```python
from build123d import *

# Parameters (mm, degrees)
SKETCH1_W                  = 63.5
SKETCH1_H                  = 60.452
BOSS_EXTRUDE1_DEPTH        = 1.27
SKETCH2_W                  = 16.51
SKETCH2_H                  = 4.826
SKETCH2_W_2                = 38.1
SKETCH2_H_2                = 8.89
SKETCH2_H_3                = 7.62
BOSS_EXTRUDE2_DEPTH        = 15.24
SKETCH3_R                  = 1.905
CUT_EXTRUDE1_DEPTH         = 25.892
SKETCH4_R                  = 3.175
CUT_EXTRUDE2_DEPTH         = 7.62
SKETCH5_W                  = 22.86
SKETCH5_H                  = 24.252018656
SKETCH5_H_2                = 1.10530733
SKETCH5_H_3                = 10.202674014
CUT_EXTRUDE3_DEPTH         = 18.78
F_8_0_199_DIAMETER_HOLE1_D = 5.0546


with BuildPart() as part:
    # Sketch1 → Boss-Extrude1 (new body, symmetric)
    with BuildSketch(Plane(origin=(0, 0, 0), x_dir=(1, 0, 0), z_dir=(0, 1, 0))):
        Rectangle(SKETCH1_W, SKETCH1_H)
    extrude(amount=BOSS_EXTRUDE1_DEPTH, both=True)

    # Sketch2 → Boss-Extrude2 (add)
    with BuildSketch(Plane(origin=(0, 1.27, 0), x_dir=(1, 0, 0), z_dir=(0, 1, 0))):
        with Locations((-23.495, 27.813)):
            Rectangle(SKETCH2_W, SKETCH2_H)
        with Locations((-23.495, -0.889)):
            Rectangle(SKETCH2_W, SKETCH2_H)
        with Locations((0, -25.781)):
            Rectangle(SKETCH2_W_2, SKETCH2_H_2)
        with Locations((0, -9.144)):
            Rectangle(SKETCH2_W_2, SKETCH2_H_3)
    extrude(amount=BOSS_EXTRUDE2_DEPTH)

    # Sketch3 → Cut-Extrude1 (cut, through all)
    with BuildSketch(Plane(origin=(0, 0, 5.334), x_dir=(-1, 0, 0), z_dir=(0, 0, -1))):
        with Locations((1.524, 4.445)):
            Circle(SKETCH3_R)
    extrude(amount=-CUT_EXTRUDE1_DEPTH, mode=Mode.SUBTRACT)

    # Sketch4 → Cut-Extrude2 (cut)
    with BuildSketch(Plane(origin=(0, 0, 5.334), x_dir=(-1, 0, 0), z_dir=(0, 0, -1))):
        with Locations((1.524, 4.445)):
            Circle(SKETCH4_R)
    extrude(amount=-CUT_EXTRUDE2_DEPTH, mode=Mode.SUBTRACT)

    # Sketch5 → Cut-Extrude3 (cut, through all)
    with BuildSketch(Plane.XZ.offset(1.27)):
        with Locations((8.89, -16.994683342)):
            Rectangle(SKETCH5_W, SKETCH5_H)
        with Locations((8.89, -29.673346335)):
            Rectangle(SKETCH5_W, SKETCH5_H_2)
        with Locations((8.89, 0.232662993)):
            Rectangle(SKETCH5_W, SKETCH5_H_3)
    extrude(amount=-CUT_EXTRUDE3_DEPTH, mode=Mode.SUBTRACT)

    # #8 (0.199) Diameter Hole1 (through all)
    with Locations(Plane(origin=(-6.35, 1.27, 1.524), x_dir=(0, 0, 1), z_dir=(0, 1, 0))):
        with Locations((0, 0), (15.875, -12.7), (-19.05, 31.75)):
            Hole(F_8_0_199_DIAMETER_HOLE1_D / 2)


solid = part.part
```
Can you work these out from the model? Positions are in its coordinate system, mm. A direction names the side the tool comes from. Give positions to 0.01 mm unless a question says otherwise; leave off trailing zeros. Loops run counter-clockwise (first coordinate to the right, second up) from the corner with the lowest first, then second, coordinate; pieces in that order, holes last. Notation, with made-up numbers: M 21.25,-10.75 L 50.25,-10.75 A19 cw 50.25,15.25 Z; hole C 87.25,82.25 d8. An arc over 180 degrees is marked long. Use CSV: the item, a comma, the result in double quotes. Start each with the question number.
1. On a 3-axis mill with a long thin cutter (end or side, diameter ignored), from which of +Z, -Z, +X, -X, +Y, -Y can I reach the whole of each face in a straight line? I mean faces 5 (the face through (-24, 9, 3.302)), 6 (the face through (-0.836, 1.346, 9.091)), 7 (the face through (-15.24, 9, -28)), 8 (the face through (19.05, 9, 9)), 9 (the face through (-19.05, 9, 9)). Say none if no direction works.
2. If we mould it in two halves opening along X, with no side actions, what happens to faces 1 (the face through (26, 0, -30.226)), 2 (the face through (-15.24, 9, 1)), 3 (the face through (-3.844, -0.018, 1.853)), 4 (the face through (-31.75, 0, -7))? For each: released by +X, released by -X, zero draft, split by the parting line, or undercut.
3. If I drill on L1, parallel to Z at x = -24, y = 5; L2, parallel to Z at x = 6.5, y = 5; L3, parallel to Y at x = 21.5, z = -6, over which ranges is the centre line in solid material (lowest first)?
4. Imagine slicing it at A-A, the plane y = 14. Write out the boundary of the cut face in (x, z).
5. For P1, Ø4, axis at y = 7.5, z = -28, coming from the +X side; P2, Ø2.5, axis at y = 12, z = 9, coming from the -X side; P3, Ø7, axis at y = 12.5, z = 27.5, coming from the +X side; P4, Ø4.5, axis at x = 25.4, z = -17.526, coming from the +Y side, each with a flat end and sliding along its axis, tell me the tip position at first contact or that it passes through.
6. Imagine slicing it at B-B, the plane z = -3. Write out the boundary of the cut face in (x, y), plus the area to 3 significant figures.
7. Imagine slicing it at D-D, the plane z = 11. Write out the boundary of the cut face in (x, y) (3 decimals).
8. Imagine slicing it at C-C, the plane x = -6.35. Write out the boundary of the cut face in (y, z), plus the area to 3 significant figures.
Response values:
1,face 5,"+X, -X, +Y"
1,face 6,"-Z"
1,face 7,"-Z, +X, +Y"
1,face 8,"+Z, -Z, +X, +Y"
1,face 9,"+Z, -X, +Y"
2,face 1,"zero draft"
2,face 2,"released by +X"
2,face 3,"undercut"
2,face 4,"released by -X"
3,L1,"-30.23 to -25.4, -1.52 to 3.3"
3,L2,"5.33 to 12.95, 21.34 to 30.23"
3,L3,"-1.27 to 1.27"
4,outline,"M -31.75,-30.23 L -15.24,-30.23 L -15.24,-25.4 L -31.75,-25.4 Z; M -31.75,-1.52 L -15.24,-1.52 L -15.24,3.3 L -31.75,3.3 Z; M -19.05,5.33 L 19.05,5.33 L 19.05,12.95 L -19.05,12.95 Z; M -19.05,21.34 L 19.05,21.34 L 19.05,30.23 L -19.05,30.23 Z"
5,P1,"x = -15.24"
5,P2,"x = -19.05"
5,P3,"x = 19.05"
5,P4,"through"
6,outline,"M -31.75,-1.27 L -2.54,-1.27 L -2.54,1.27 L -31.75,1.27 Z; M 20.32,-1.27 L 31.75,-1.27 L 31.75,1.27 L 20.32,1.27 Z"
6,area,"103 mm^2"
7,outline,"M -31.75,-1.27 L 31.75,-1.27 L 31.75,1.27 L 19.05,1.27 L 19.05,16.51 L -19.05,16.51 L -19.05,1.27 L -31.75,1.27 Z; hole C -1.524,4.445 d6.35"
8,outline,"M -1.27,-30.23 L 1.27,-30.23 L 1.27,-1 L -1.27,-1 Z; M -1.27,4.05 L 1.27,4.05 L 1.27,5.33 L 16.51,5.33 L 16.51,12.95 L 1.27,12.95 L 1.27,21.34 L 16.51,21.34 L 16.51,30.23 L -1.27,30.23 Z"
8,area,"392 mm^2"
